Design review of the part built by this model. Coordinates are the model's own, in mm. Face numbers are marked on the shaded views. A direction names the side the tool comes from. Coordinates: 2 decimals unless noted, no trailing zeros. Order: outer loops, then holes, each group sorted by start corner. A loop starts at its lowest first (then second) coordinate and runs counter-clockwise, first axis right, second up. Notation, with made-up numbers: M 61.25,2 L 111.25,2 A14 ccw 111.25,11 Z; hole C 18.25,23 d8. An arc over 180 degrees is marked long. Answer in a Markdown table with one row per item.
from build123d import *

# Parameters (mm, degrees)
SKETCH_1_R          = 26
EXTRUDE_1_DEPTH     = 23.65
SKETCH_2_R          = 19.9
EXTRUDE_2_DEPTH     = 36.05
CUT_EXTRUDE_1_DEPTH = 36.05
SKETCH_4_R          = 1.25
CUT_EXTRUDE_2_DEPTH = 2


with BuildPart() as part:
    # 草图1 → 凸台-拉伸1 (new body)
    with BuildSketch(Plane(origin=(0, 0, 0), x_dir=(1, 0, 0), z_dir=(0, 1, 0))):
        Circle(SKETCH_1_R)
    extrude(amount=EXTRUDE_1_DEPTH)

    # 草图2 → 凸台-拉伸2 (add)
    with BuildSketch(Plane.XZ):
        Circle(SKETCH_2_R)
    extrude(amount=-EXTRUDE_2_DEPTH)

    # 草图3 → 切除-拉伸1 (cut)
    with BuildSketch(Plane.XZ):
        with BuildLine():
            Line((23.966938911, 10.078980068), (23.966938911, -10.078980068))
            ThreePointArc((23.966938911, -10.078980068), (26, 0), (23.966938911, 10.078980068))
        make_face()
    extrude(amount=-CUT_EXTRUDE_1_DEPTH, mode=Mode.SUBTRACT)

    # 草图4 → 切除-拉伸2 (cut)
    with BuildSketch(Plane.XZ):
        with Locations((-14.000714267, -14.000714267)):
            Circle(SKETCH_4_R)
        with Locations((14.000714267, 14.000714267)):
            Circle(SKETCH_4_R)
    extrude(amount=-CUT_EXTRUDE_2_DEPTH, mode=Mode.SUBTRACT)


solid = part.part
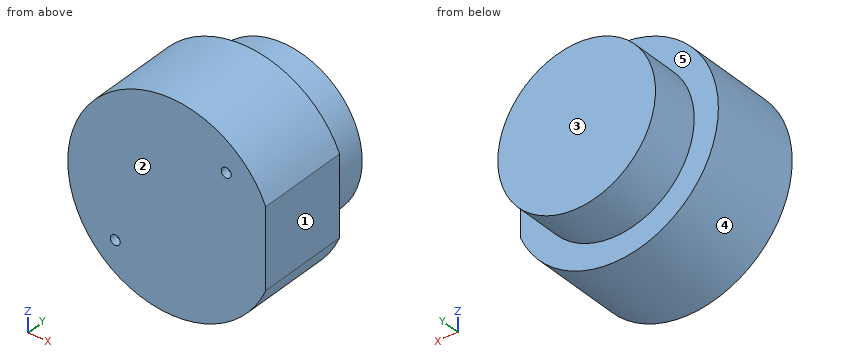
(1) For line 1 along Y through (x, z) = (16, 13); line 2 along X through (y, z) = (31, 7); line 3 along Z through (x, y) = (15, 7), list the stretches that pass through material, from the lowest coordinate up. Write a range as from..to.
Return value:
| item | result |
|---|---|
| line 1 | y = 0..23.65 |
| line 2 | x = -18.63..18.63 |
| line 3 | z = -21.24..21.24 |
(2) Add section C-C, the plane y = 5. Give the boundary of the cut face in (x, z), and give its area (3 significant figures).
Return value:
| item | result |
|---|---|
| outline | M 23.97,-10.08 L 23.97,10.08 A26 ccw long Z |
| area | 2,100 mm2 |
(3) Add section D-D, the plane y = 32.5. Give the boundary of the cut face in (x, z).
Return value:
| item | result |
|---|---|
| outline | C 0,0 d39.8 |
(4) For the marked faces 4 and 5, list the 3-axis set-ups (+Z, -Z, +X, -X, +Y, -Y) from which the entire face can be reached by the end or side of a thin tool; tool diameter is ignored.
Return value:
| item | result |
|---|---|
| face 4 | +Y, -Y |
| face 5 | +Y |
(5) Add section B-B, the plane x = 0. Give the boundary of the cut face in (y, z), and give its area (3 significant figures).
Return value:
| item | result |
|---|---|
| outline | M 0,-26 L 23.65,-26 L 23.65,-19.9 L 36.05,-19.9 L 36.05,19.9 L 23.65,19.9 L 23.65,26 L 0,26 Z |
| area | 1,720 mm2 |
(6) Draft analysis for pull direction Y (two halves, no side actions). For the marked faces 1, 2 and 3, state which applies: pulls with the +Y half, pulls with the -Y half, needs draft (parallel to the pull), parting line crosses it, or undercut.
Return value:
| item | result |
|---|---|
| face 1 | needs draft |
| face 2 | pulls with the -Y half |
| face 3 | pulls with the +Y half |
(7) Insertion check: pin 1 Ø1 at (x, z) = (-19, 12) entering from +Y; pin 2 Ø4 at (x, y) = (-15, 16.5) entering from +Z; pin 3 Ø2 at (x, z) = (14, 14) entering from -Y. Each pin has a flat end and moves straight along its axis. Give the tip position at first contact, or say it passes through.
Return value:
| item | result |
|---|---|
| pin 1 | stops at y = 23.65 |
| pin 2 | stops at z = 22.52 |
| pin 3 | stops at y = 2 |
(8) Add section A-A, the plane z = 0. Give the boundary of the cut face in (x, y).
Return value:
| item | result |
|---|---|
| outline | M -26,0 L 23.97,0 L 23.97,23.65 L 19.9,23.65 L 19.9,36.05 L -19.9,36.05 L -19.9,23.65 L -26,23.65 Z |
